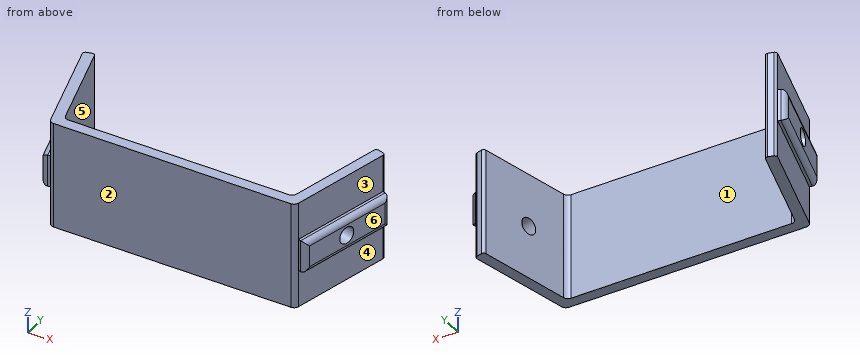
```python
from build123d import *

# Parameters (mm, degrees)
F1_DEPTH = 20
F2_W     = 18.732673012
F2_H     = 6
F3_DEPTH = 1.5
F4_W     = 18.732673012
F4_H     = 6
F5_DEPTH = 1.5
F6_R     = 1.55
F7_DEPTH = 12.5
F8_R     = 1.55
F9_DEPTH = 12.5
F10_R    = 1


with BuildPart() as f1:
    # F0 (on Top) → F1 (new body)
    with BuildSketch(Plane.XY):
        with BuildLine():
            ThreePointArc((-0.1985988383, 0.7411809549), (0.158565559, 0.2066466597), (0.767326988, 0))
            Line((0.767326988, 0), (44.232673012, 0))
            ThreePointArc((44.232673012, 0), (44.841434441, 0.2066466597), (45.1985988383, 0.7411809549))
            Line((45.1985988383, 0.7411809549), (50.0469713795, 18.8355536126))
            ThreePointArc((50.0469713795, 18.8355536126), (49.9970211682, 19.2149631352), (49.6934179889, 19.4479260483))
            Line((49.6934179889, 19.4479260483), (48.7274921626, 19.7067450934))
            ThreePointArc((48.7274921626, 19.7067450934), (48.3480826401, 19.6567948822), (48.1151197269, 19.3531917028))
            Line((48.1151197269, 19.3531917028), (43.6639448624, 2.7411809549))
            ThreePointArc((43.6639448624, 2.7411809549), (43.3067804651, 2.2066466597), (42.6980190361, 2))
            Line((42.6980190361, 2), (2.3019809639, 2))
            ThreePointArc((2.3019809639, 2), (1.6932195349, 2.2066466597), (1.3360551376, 2.7411809549))
            Line((1.3360551376, 2.7411809549), (-3.1151197269, 19.3531917028))
            ThreePointArc((-3.1151197269, 19.3531917028), (-3.3480826401, 19.6567948822), (-3.7274921626, 19.7067450934))
            Line((-3.7274921626, 19.7067450934), (-4.6934179889, 19.4479260483))
            ThreePointArc((-4.6934179889, 19.4479260483), (-4.9970211682, 19.2149631352), (-5.0469713795, 18.8355536126))
            Line((-5.0469713795, 18.8355536126), (-0.1985988383, 0.7411809549))
        make_face()
    extrude(amount=F1_DEPTH)

    # F2 (on face) → F3 (join)
    with BuildSketch(Plane(origin=(41.9855715851, -11.25, 0), x_dir=(0.2588190451, 0.9659258263, 0), z_dir=(0.9659258263, -0.2588190451, 0))):
        with Locations((21.7805205236, 10)):
            Rectangle(F2_W, F2_H)
    extrude(amount=F3_DEPTH)

    # F4 (on face) → F5 (join)
    with BuildSketch(Plane(origin=(0, 0, 0), x_dir=(0.2588190451, -0.9659258263, 0), z_dir=(-0.9659258263, -0.2588190451, 0))):
        with Locations((-10.133663494, 10)):
            Rectangle(F4_W, F4_H)
    extrude(amount=F5_DEPTH)

    # F6 (on face) → F7 (cut, symmetric)
    with BuildSketch(Plane(origin=(0, 0, 0), x_dir=(0.2588190451, -0.9659258263, 0), z_dir=(-0.9659258263, -0.2588190451, 0))):
        with Locations((-10, 10)):
            Circle(F6_R)
    extrude(amount=F7_DEPTH, both=True, mode=Mode.SUBTRACT)

    # F8 (on face) → F9 (cut, symmetric)
    with BuildSketch(Plane(origin=(41.9855715851, -11.25, 0), x_dir=(0.2588190451, 0.9659258263, 0), z_dir=(0.9659258263, -0.2588190451, 0))):
        with Locations((21.6468570296, 10)):
            Circle(F8_R)
    extrude(amount=F9_DEPTH, both=True, mode=Mode.SUBTRACT)

    # F10
    f10_edges = [f1.edges().sort_by_distance(p)[0] for p in [
        (-1.647488, 0.352952, 10),
        (-4.071674, 9.400139, 7),
        (-4.071674, 9.400139, 13),
        (-6.49586, 18.447325, 10),
        (51.49586, 18.447325, 10),
        (49.071674, 9.400139, 7),
        (49.071674, 9.400139, 13),
        (46.647488, 0.352952, 10),
    ]]
    fillet(f10_edges, radius=F10_R)


solid = f1.part
```
Here's how the part is built. I have some questions about the finished solid (model axes, mm). Face numbers are marked on the shaded views. A direction names the side the tool comes from. Round coordinates to 2 decimals unless told otherwise and drop trailing zeros. Loops run counter-clockwise (first coordinate to the right, second up) from the corner with the lowest first, then second, coordinate; pieces in that order, holes last. Notation, with made-up numbers: (17.25, 72) -> (71.25, 72) arc R10 cw to (71.25, 85) -> close; hole circle Ø5 at (31.5, -20). An arc over 180 degrees is marked (long way). Answer as CSV lines item,"result". Start each with the question number.
1. Imagine slicing it at A-A on z = 14. Write out the boundary of the cut face in (x, y).
2. I need wall thicknesses on probe 1 along Y at (x, z) = (40.5, 3.75); probe 2 along Z at (x, y) = (46.5, 5.25); probe 3 along X at (y, z) = (10.75, 17.25). Which ranges of each line are inside material? Lowest first, please. Write a range as from..to.
3. If we mould it in two halves opening along X, with no side actions, what happens to the marked faces 1, 2 and 3? For each: pulls with the +X half, pulls with the -X half, needs draft (parallel to the pull), parting line crosses it, or undercut.
4. For the marked faces 4, 5 and 6, which set-ups out of +Z, -Z, +X, -X, +Y, -Y let a thin tool reach every point of the face, with its end or its side?
5. Imagine slicing it at B-B on x = 30.5. Write out the boundary of the cut face in (y, z).
6. I'm going to push flat-ended pins straight in: P1, Ø10, axis at y = 13.5, z = 16, coming from the +X side; P2, Ø1.5, axis at x = 33, z = 12.5, coming from the +Y side; P3, Ø10, axis at y = 2.5, z = 15.5, coming from the -X side. Where does each tip first touch, or does it pass through?
Solution:
1,outline,"(-5.05, 18.84) -> (-0.2, 0.74) arc R1 ccw to (0.77, 0) -> (44.23, 0) arc R1 ccw to (45.2, 0.74) -> (50.05, 18.84) arc R0.5 ccw to (49.69, 19.45) -> (48.73, 19.71) arc R0.5 ccw to (48.12, 19.35) -> (43.66, 2.74) arc R1 cw to (42.7, 2) -> (2.3, 2) arc R1 cw to (1.34, 2.74) -> (-3.12, 19.35) arc R0.5 ccw to (-3.73, 19.71) -> (-4.69, 19.45) arc R0.5 ccw to start"
2,probe 1,"0..2"
2,probe 2,"7..13"
2,probe 3,"-2.88..-0.81, 45.81..47.88"
3,face 1,"undercut"
3,face 2,"needs draft"
3,face 3,"pulls with the +X half"
4,face 4,"-Z, +X, -Y"
4,face 5,"+Z, -Z, +Y"
4,face 6,"+Z, -Z, +X, -Y"
5,outline,"(0, 0) -> (2, 0) -> (2, 20) -> (0, 20) -> close"
6,P1,"x = 51.02"
6,P2,"y = 2"
6,P3,"x = -3.21"
